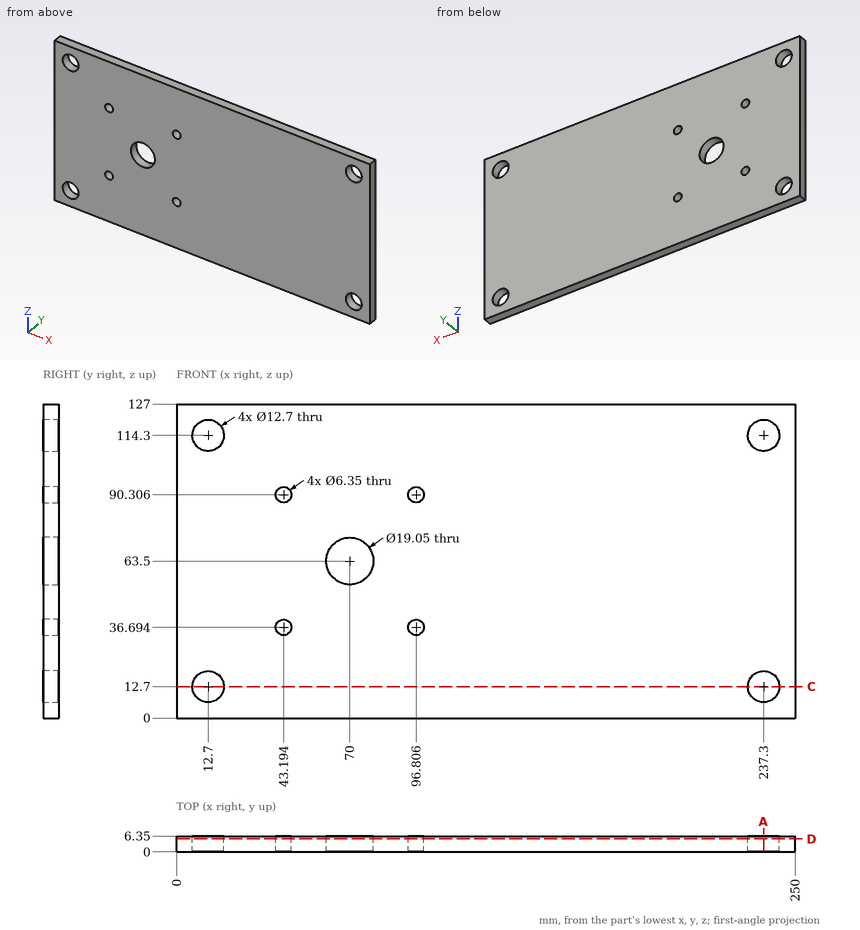
Part print with two shaded views. Sizes in mm from the minimum x, y, z corner. Give positions to 0.01 mm unless a question says otherwise; leave off trailing zeros. Loops run counter-clockwise (first coordinate to the right, second up) from the corner with the lowest first, then second, coordinate; pieces in that order, holes last. Notation, with made-up numbers: (75, -39) - (93, -39) arc R34 ccw to (93, -8) - close; hole circle Ø8 at (5, 4.25). An arc over 180 degrees is marked (long way). Put each result on its own line as item: value.
Q1. Probe line 1 along X through (y, z) = (1, 90); line 2 along X through (y, z) = (2, 114.3); line 3 along X through (y, z) = (4.75, 63.5) (1 decimal). List the from-to ranges inside material, lowest first.
Filled in:
line 1: x = 0 to 40.03, 46.35 to 93.65, 99.97 to 250
line 2: x = 0 to 6.35, 19.05 to 230.95, 243.65 to 250
line 3: x = 0 to 60.5, 79.5 to 250
Q2. Slice it at A-A (x = 237.3). Give the cut face in (y, z), plus the area to 3 significant figures.
Filled in:
outline: (0, 0) - (6.35, 0) - (6.35, 6.35) - (0, 6.35) - close; (0, 19.05) - (6.35, 19.05) - (6.35, 107.95) - (0, 107.95) - close; (0, 120.65) - (6.35, 120.65) - (6.35, 127) - (0, 127) - close
area: 645 mm²
Q3. Slice it at C-C (z = 12.7). Give the cut face in (x, y), plus the area to 3 significant figures.
Filled in:
outline: (0, 0) - (6.35, 0) - (6.35, 6.35) - (0, 6.35) - close; (19.05, 0) - (230.95, 0) - (230.95, 6.35) - (19.05, 6.35) - close; (243.65, 0) - (250, 0) - (250, 6.35) - (243.65, 6.35) - close
area: 1,430 mm²
Q4. Slice it at D-D (y = 5.25). Give the number of separate pieces and of enclosed holes in the cut face, plus the area to 3 significant figures.
Filled in:
separate pieces: 1
enclosed holes: 9
area: 30,800 mm²
Q5. Flat gauge pins, fed straight in: pin 1 (1 mm diameter, centred on x = 183, y = 1, fed in from -Z); pin 2 (7.5 mm diameter, centred on x = 237.3, z = 114.3, fed in from +Y). Where does each tip first touch, or does it go through?
Filled in:
pin 1: stops at z = 0
pin 2: passes through
